Input: part model. Units: mm. Frame: model coordinates. A direction names the side the tool comes from. Give positions to 0.01 mm unless a question says otherwise; leave off trailing zeros. Loops run counter-clockwise (first coordinate to the right, second up) from the corner with the lowest first, then second, coordinate; pieces in that order, holes last. Notation, with made-up numbers: M 80,19.25 L 130,19.25 A11 cw 130,32.25 Z; hole C 78.25,-32 d6. An arc over 180 degrees is marked long. Answer as a JSON object with one key per item and string values. Group by question number.
1) Section query A-A on z = 15. Return loops of the section in (x, y).
2) Section query C-C on z = 8. Return loops of the section in (x, y), plus the area to 3 significant figures.
3) Draft query along X for faces 1 (the flat face through (-15, -11.3, 6.2)), 2 (the cylindrical face through (-8.7, -1, 8.9)), 3 (the flat face through (-7, -13, 8)), 4 (the flat face through (0, -11.3, 6.2)). Return one class per face: +X half, -X half, draft (parallel to the pull), parting line (faces both ways), or undercut.
4) Section query D-D on x = -14. Return loops of the section in (y, z), plus the area to 3 significant figures.
5) Ray query, L1, parallel to Y at x = -6, z = 9.5; L2, parallel to X at y = -1.05, z = 8; L3, parallel to Z at x = -7.5, y = -0.7. Return the intervals inside material, ascending.
6) Access query for faces 5 (the flat face through (-7, -11, 9)), 6 (the flat face through (-5.7, 0, 8.1)). Directions: +Z, -Z, +X, -X, +Y, -Y. A direction counts if a zero-diameter tool reaches every point of the face in a straight line with its end or side. Return the directions, or none.
7) First-contact query: P1, Ø2.5, axis at x = -10.5, y = -8.5, coming from the +Z side. Flat tip, straight axial feed; report the tip coordinate or a pass-through.
8) Section query B-B on x = -7.5. Return loops of the section in (y, z).
from build123d import *

# Parameters (mm, degrees)
BOSS_EXTRUDE1_DEPTH = 15
CUT_EXTRUDE1_REACH  = 15
SKETCH2_R           = 1.5


with BuildPart() as part:
    # Sketch1 → Boss-Extrude1 (new body)
    with BuildSketch(Plane(origin=(0, 0, 0), x_dir=(0, 0, -1), z_dir=(1, 0, 0))):
        Polygon((0, 0), (0, -13), (-16, -13), (-16, -11), (-2, -11), (-2, -2), (-16, -2), (-16, 0), align=None)
    extrude(amount=-BOSS_EXTRUDE1_DEPTH)

    # Sketch2 → Cut-Extrude1 (cut, up to next)
    with BuildSketch(Plane(origin=(0, 0, 0), x_dir=(1, 0, 0), z_dir=(0, 1, 0)), mode=Mode.PRIVATE) as cut_extrude1_sk1:
        with Locations((-7.5, -8)):
            Circle(SKETCH2_R)
    cut_extrude1_tool1 = extrude(cut_extrude1_sk1.sketch, amount=-CUT_EXTRUDE1_REACH, mode=Mode.PRIVATE) & part.part
    add(cut_extrude1_tool1.solids().sort_by_distance((-7.5, 0, 8))[0], mode=Mode.SUBTRACT)


solid = part.part
Output:
{
 "1": {"outline": "M -15,-13 L 0,-13 L 0,-11 L -15,-11 Z; M -15,-2 L 0,-2 L 0,0 L -15,0 Z"},
 "2": {"outline": "M -15,-13 L 0,-13 L 0,-11 L -15,-11 Z; M -15,-2 L -9,-2 L -9,0 L -15,0 Z; M -6,-2 L 0,-2 L 0,0 L -6,0 Z", "area": "54.0 mm^2"},
 "3": {"face 1": "-X half", "face 2": "undercut", "face 3": "draft", "face 4": "+X half"},
 "4": {"outline": "M -13,0 L 0,0 L 0,16 L -2,16 L -2,2 L -11,2 L -11,16 L -13,16 Z", "area": "82.0 mm^2"},
 "5": {"L1": "y = -13 to -11, -2 to 0", "L2": "x = -15 to -9, -6 to 0", "L3": "z = 0 to 6.5, 9.5 to 16"},
 "6": {"face 5": "+Z, +X, -X", "face 6": "+Z, -Z, +X, -X, +Y"},
 "7": {"P1": "stops at z = 2"},
 "8": {"outline": "M -13,0 L 0,0 L 0,6.5 L -2,6.5 L -2,2 L -11,2 L -11,16 L -13,16 Z; M -2,9.5 L 0,9.5 L 0,16 L -2,16 Z"}
}
